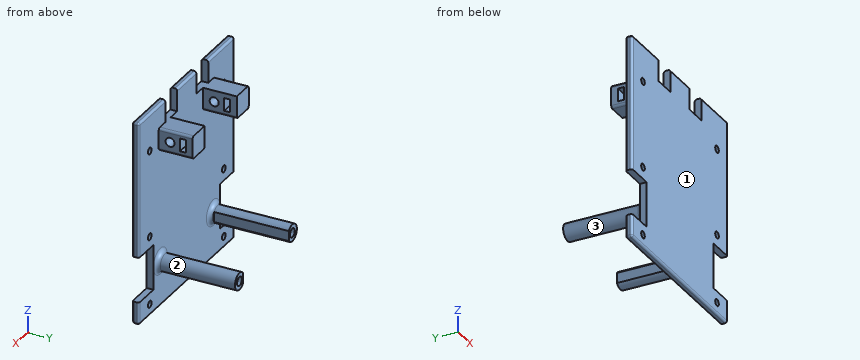
Autodesk Inventor part; units mm, degrees
ref_plane "YZ Plane" through (0, 0, 0) normal (1, 0, 0) x (0, 1, 0)
ref_plane "XZ Plane" through (0, 0, 0) normal (0, 1, 0) x (-1, 0, 0)
ref_plane "XY Plane" through (0, 0, 0) normal (0, 0, 1) x (1, 0, 0)
sketch "Эскиз1" plane through (0, 0, 0) normal (0, 1, 0) x (-1, 0, 0)
  line L0 (6, 63) -> (-74, 63)
  line L1 (-74, 63) -> (-74, -27)
  line L2 (-74, -27) -> (6, -27)
  line L3 (6, -27) -> (6, 63)
  line L4 (-3, 8.202) -> (-65, 8.202)
  line L5 (-65, 8.202) -> (-65, -22)
  line L6 (-65, -22) -> (-3, -22)
  line L7 (-3, -22) -> (-3, 8.202)
  circle A0 centre (-3, 8.202) radius 1.5
  circle A1 centre (-3, -22) radius 1.5
  circle A2 centre (-65, 8.202) radius 1.5
  circle A3 centre (-65, -22) radius 1.5
  circle A4 centre (-3, 46.5) radius 1.5
  circle A5 centre (-65, 46.5) radius 1.5
  point P0 (0, 0)
  dimension "d0" = 80
  dimension "d1" = 90
  dimension "d2" = 30.202
  dimension "d3" = 5
  dimension "d4" = 62
  dimension "d5" = 9
  dimension "d6" = 3
  dimension "d7" = 3
  dimension "d8" = 3
  dimension "d9" = 3
  dimension "d10" = 3
  dimension "d11" = 9
  dimension "d12" = 16.5
  dimension "d13" = 3
  dimension "d14" = 16.5
  dimension "d15" = 9
extrude "Выдавливание1" add sketch "Эскиз1" along normal blind 3 contours L3 L2 L1 L0 | L4 A0 L7 A1 L6 A3 L5 A2
sketch "Эскиз2" plane through (0, 3, 0) normal (0, 1, 0) x (1, 0, 0)
  line L0 (10.5, -53) -> (20.5, -53)
  line L1 (20.5, -53) -> (20.5, -43)
  line L2 (20.5, -43) -> (10.5, -43)
  line L3 (10.5, -43) -> (10.5, -53)
  line L4 (47.5, -53) -> (57.5, -53)
  line L5 (57.5, -53) -> (57.5, -43)
  line L6 (57.5, -43) -> (47.5, -43)
  line L7 (47.5, -43) -> (47.5, -53)
  line L8 (-6, -63) -> (74, -63)
  line L9 (-6, 27) -> (-6, -63)
  point P0 (0, 0)
  point P1 (15.5, -53)
  point P2 (20.5, -48)
  dimension "d18" = 10
  dimension "d19" = 10
  dimension "d20" = 10
  dimension "d21" = 27
  dimension "d23" = 10
  dimension "d24" = 16.5
extrude "Выдавливание2" add sketch "Эскиз2" along normal blind 15
sketch "Эскиз3" plane through (57.5, 3, 53) normal (1, 0, 0) x (0, 0, -1)
  line L0 (2.15, 12) -> (7.85, 12)
  line L1 (7.85, 12) -> (7.85, 9.4)
  line L2 (7.85, 9.4) -> (2.15, 9.4)
  line L3 (2.15, 9.4) -> (2.15, 12)
  circle A0 centre (5, 5) radius 2
  line L4 (0, 15) -> (10, 15)
  line L5 (10, 0) -> (10, 15)
  point P0 (53, -3)
  dimension "d27" = 4
  dimension "d28" = 5.7
  dimension "d29" = 2.6
  dimension "d30" = 3
  dimension "d31" = 2.15
  dimension "d32" = 10
  dimension "d33" = 5
extrude "Выдавливание3" cut sketch "Эскиз3" against normal blind 78
fillet "Сопряжение2" radius 1 12 edges at (74, 0, 18) (74, 3, 18) (34, 0, -27) (74, 1.5, -27) (34, 3, -27) (-6, 3, 18) (-6, 0, 18) (34, 3, 63) (34, 0, 63) (-6, 1.5, 63) (74, 1.5, 63) (-6, 1.5, -27)
sketch "Эскиз6" plane through (0, 3, 0) normal (0, 1, 0) x (1, 0, 0)
  line L0 (14, 16) -> (-1, 16)
  line L1 (-1, 16) -> (-1, -2)
  line L2 (-1, -2) -> (14, -2)
  line L3 (14, -2) -> (14, 16)
  line L4 (73, 27) -> (-5, 27)
  line L5 (-6, 26) -> (-6, -62)
  line L6 (69, 16) -> (54, 16)
  line L7 (54, 16) -> (54, -2)
  line L8 (54, -2) -> (69, -2)
  line L9 (69, -2) -> (69, 16)
  line L10 (74, -62) -> (74, 26)
  circle A0 centre (11.85, 7) radius 2
  circle A1 centre (11.85, 7) radius 3.75
  circle A2 centre (56.15, 7) radius 2
  circle A3 centre (56.15, 7) radius 3.75
  point P0 (0, 0)
  dimension "d38" = 15
  dimension "d39" = 18
  dimension "d40" = 11
  dimension "d41" = 5
  dimension "d42" = 15
  dimension "d43" = 18
  dimension "d44" = 11
  dimension "d45" = 5
  dimension "d49" = 4
  dimension "d50" = 7.5
  dimension "d51" = 4
  dimension "d52" = 7.5
  dimension "d54" = 44.3
  dimension "d56" = 17.85
extrude "Выдавливание4" add sketch "Эскиз6" along normal blind 35 contours A1 L3 | L3 A1 | A3 L7 | L7 A3
fillet "Сопряжение4" radius 2 2 edges at (8.1, 3, -7) (52.4, 3, -7)
sketch "Эскиз7" plane through (11.85, 38, -7) normal (0, 1, 0) x (1, 0, 0)
  circle A0 centre (0, 0) radius 3.75
  line L0 (3, 2.25) -> (3, -2.25)
  circle A1 centre (44.3, 0) radius 3.75
  line L1 (41.3, 2.25) -> (41.3, -2.25)
  point P0 (-11.85, -7)
extrude "Выдавливание5" cut sketch "Эскиз7" against normal blind 33 contours A0 L0 | L1 A1 picked at (3.1367, -0.52) picked at (41.1633, -0.52)
fillet "Сопряжение5" radius 1 6 edges at (10.5, 10.5, 43) (20.5, 10.5, 43) (47.5, 10.5, 43) (57.5, 10.5, 43) (57.5, 10.5, 53) (10.5, 10.5, 53)
sketch "Эскиз12" plane through (0, 3, 0) normal (0, 1, 0) x (1, 0, 0)
  line L0 (73, -63) -> (-5, -63)
  line L1 (11.5, -53) -> (20.5, -53)
  line L2 (16, -53) -> (26, -53)
  line L3 (26, -53) -> (26, -63)
  line L4 (26, -63) -> (16, -63)
  line L5 (16, -63) -> (16, -53)
  line L6 (47.5, -53) -> (56.5, -53)
  line L7 (52, -53) -> (42, -53)
  line L8 (42, -53) -> (42, -63)
  line L9 (42, -63) -> (52, -63)
  line L10 (52, -63) -> (52, -53)
  point P0 (0, 0)
extrude "Выдавливание9" cut sketch "Эскиз12" against normal blind 10
sketch "Эскиз14" plane through (0, 3, 0) normal (0, 1, 0) x (1, 0, 0)
  circle A0 centre (11.85, 7) radius 5.75
  line L0 (6.1, 7) -> (6.1, -3)
  line L1 (6.1, 17) -> (-6, 17)
  line L2 (-6, 17) -> (-6, -3)
  line L3 (-6, -3) -> (6.1, -3)
  line L4 (6.1, -3) -> (6.1, 17)
  arc A1 (53.15, 4.75) -> (53.15, 9.25) centre (56.15, 7) ccw
  circle A2 centre (56.15, 7) radius 5.75
  line L5 (61.9, 7) -> (61.9, 17)
  line L6 (61.9, 17) -> (74, 17)
  line L7 (74, 17) -> (74, -3)
  line L8 (74, -3) -> (61.9, -3)
  line L9 (61.9, -3) -> (61.9, 17)
  point P0 (0, 0)
extrude "Выдавливание11" cut sketch "Эскиз14" against normal blind 10 contours L0 L3 L2 L1 L4 | L5 L6 L7 L8 L9
properties part number "kreplenie_dribler_V4"
Could you check a few things on this model? Use its own coordinates, in mm. Face numbers are marked on the shaded views. Give positions to 0.01 mm unless a question says otherwise; leave off trailing zeros. Order: outer loops, then holes, each group sorted by start corner. A loop starts at its lowest first (then second) coordinate and runs counter-clockwise, first axis right, second up.
1. Suppose I cut it at C-C (z = -22). Write out the boundary of the cut face in (x, y).
Answers below:
outline: (-6, 1) arc R1 ccw to (-5, 0) - (1.5, 0) - (1.5, 3) - (-5, 3) arc R1 ccw to (-6, 2) - close; (4.5, 0) - (63.5, 0) - (63.5, 3) - (4.5, 3) - close; (66.5, 0) - (73, 0) arc R1 ccw to (74, 1) - (74, 2) arc R1 ccw to (73, 3) - (66.5, 3) - close
2. For pin 1 (6.5 mm diameter, centred on x = 53, z = 48.5, fed in from +Y); pin 2 (3 mm diameter, centred on x = 56.5, z = -7, fed in from +Y); pin 3 (10 mm diameter, centred on y = 13.5, z = 50, fed in from +X), each with a flat end and sliding along its axis, tell me the tip position at first contact or that it passes through.
Answers below:
pin 1: stops at y = 18
pin 2: stops at y = 3
pin 3: stops at x = 57.5
3. Suppose I cut it at B-B (y = 29). Write out the boundary of the cut face in (x, z), plus the area to 3 significant figures.
Answers below:
outline: (14.85, -9.25) - (14.85, -4.75) arc R3.75 ccw (long way) to start; (53.15, -9.25) arc R3.75 ccw (long way) to (53.15, -4.75) - close; hole circle Ø4 at (11.85, -7); hole circle Ø4 at (56.15, -7)
area: 58.6 mm2
4. Suppose I cut it at D-D (x = 3). Write out the boundary of the cut face in (y, z), plus the area to 3 significant figures.
Answers below:
outline: (0, -26) arc R1 ccw to (1, -27) - (2, -27) arc R1 ccw to (3, -26) - (3, -23.5) - (0, -23.5) - close; (0, -20.5) - (3, -20.5) - (3, -17) - (0, -17) - close; (0, 3) - (3, 3) - (3, 6.7) - (0, 6.7) - close; (0, 9.7) - (3, 9.7) - (3, 45) - (0, 45) - close; (0, 48) - (3, 48) - (3, 62) arc R1 ccw to (2, 63) - (1, 63) arc R1 ccw to (0, 62) - close
area: 182 mm2
5. I need wall thicknesses on L1, parallel to X at y = 1.5, z = -22; L2, parallel to X at y = 24.5, z = -7; L3, parallel to Y at x = 53, z = 48. Which ranges of each line are inside material? Lowest first, please.
Answers below:
L1: x = -6 to 1.5, 4.5 to 63.5, 66.5 to 74
L2: x = 8.1 to 9.85, 13.85 to 14.85, 53.15 to 54.15, 58.15 to 59.9
L3: y = 0 to 6, 10 to 12.4, 15 to 18
6. Thinking about a two-plate mould opening in X: for the marked faces 1, 2 and 3, which applies, +X half, -X half, draft (parallel to the pull), parting line (faces both ways), or undercut?
Answers below:
face 1: draft
face 2: undercut
face 3: undercut
7. Suppose I cut it at A-A (y = 8). Write out the boundary of the cut face in (x, z).
Answers below:
outline: (10.5, 44) arc R1 ccw to (11.5, 43) - (19.5, 43) arc R1 ccw to (20.5, 44) - (20.5, 46) - (10.5, 46) - close; (10.5, 50) - (20.5, 50) - (20.5, 53) - (11.5, 53) arc R1 ccw to (10.5, 52) - close; (14.85, -9.25) - (14.85, -4.75) arc R3.75 ccw (long way) to start; (47.5, 44) arc R1 ccw to (48.5, 43) - (56.5, 43) arc R1 ccw to (57.5, 44) - (57.5, 46) - (47.5, 46) - close; (47.5, 50) - (57.5, 50) - (57.5, 52) arc R1 ccw to (56.5, 53) - (47.5, 53) - close; (53.15, -9.25) arc R3.75 ccw (long way) to (53.15, -4.75) - close; hole circle Ø4 at (11.85, -7); hole circle Ø4 at (56.15, -7)
